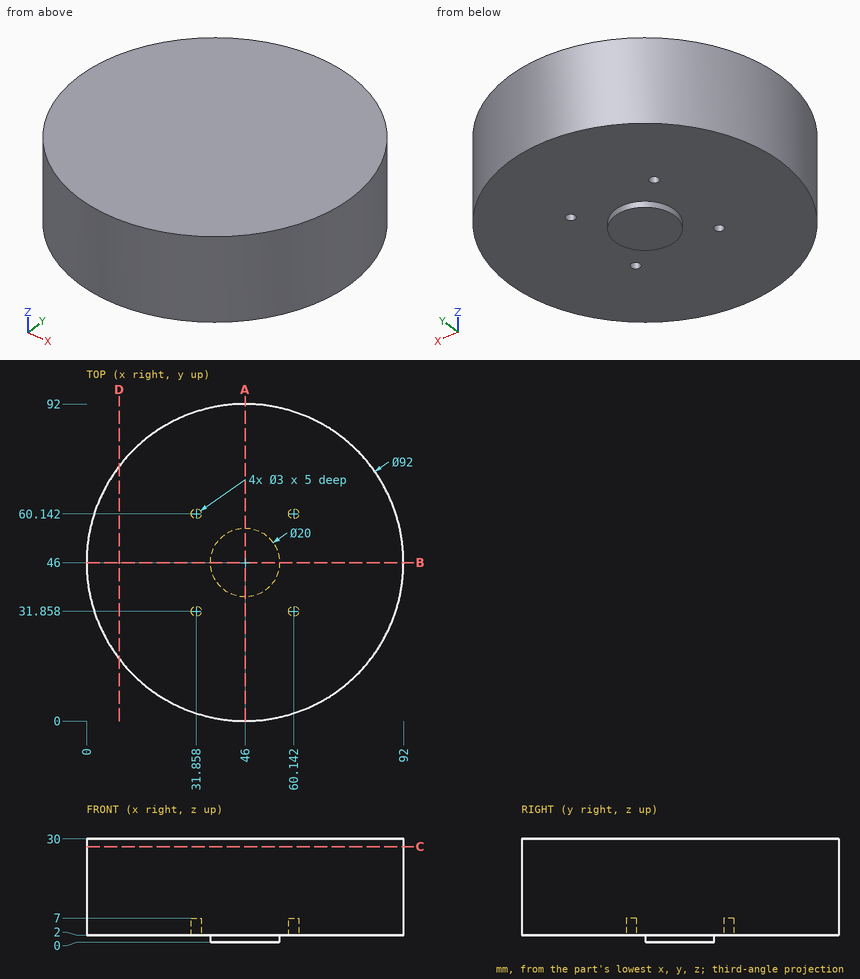
Design review of the part shown in the three views and the two pictorial views. Dimensions are in mm from the part's minimum x, y and z. Round coordinates to 2 decimals unless told otherwise and drop trailing zeros. Order: outer loops, then holes, each group sorted by start corner. A loop starts at its lowest first (then second) coordinate and runs counter-clockwise, first axis right, second up. Notation, with made-up numbers: M 62,49.25 L 79,49.25 A21 ccw 79,61.25 Z; hole C 66,44.5 d11. An arc over 180 degrees is marked long. Put each result on its own line as item: value.
Q1. Consider section A-A (x = 46). State the section outline as (y, z) points.
Reported:
outline: M 0,2 L 36,2 L 36,0 L 56,0 L 56,2 L 92,2 L 92,30 L 0,30 Z
Q2. Insertion check: pin 1 Ø10 at (x, z) = (21, 18.5) entering from +Y; pin 2 Ø5 at (y, z) = (14, 11) entering from -X (1 decimal); pin 3 Ø0.9 at (x, y) = (59.5, 31.5) entering from -Z. Each pin has a flat end and moves straight along its axis. Give the tip position at first contact, or say it passes through.
Reported:
pin 1: y = 87.42
pin 2: x = 10.7
pin 3: z = 7
Q3. To check wall thickness, follow line 1 (Y direction, x = 59, z = 3.25) (1 decimal); line 2 (Z direction, x = 45, y = 14); line 3 (Y direction, x = 23, z = 24.25). State the ranges of each line that lie inside material, in increasing order.
Reported:
line 1: 1.9 to 30.9, 32.8 to 59.2, 61.1 to 90.1
line 2: 2 to 30
line 3: 6.16 to 85.84
Q4. Consider section D-D (x = 9.5). State the section outline as (y, z) points.
Reported:
outline: M 18,2 L 74,2 L 74,30 L 18,30 Z
Q5. Consider section C-C (z = 27.75). State the section outline as (x, y) points, and give its area (3 significant figures).
Reported:
outline: C 46,46 d92
area: 6,650 mm²
